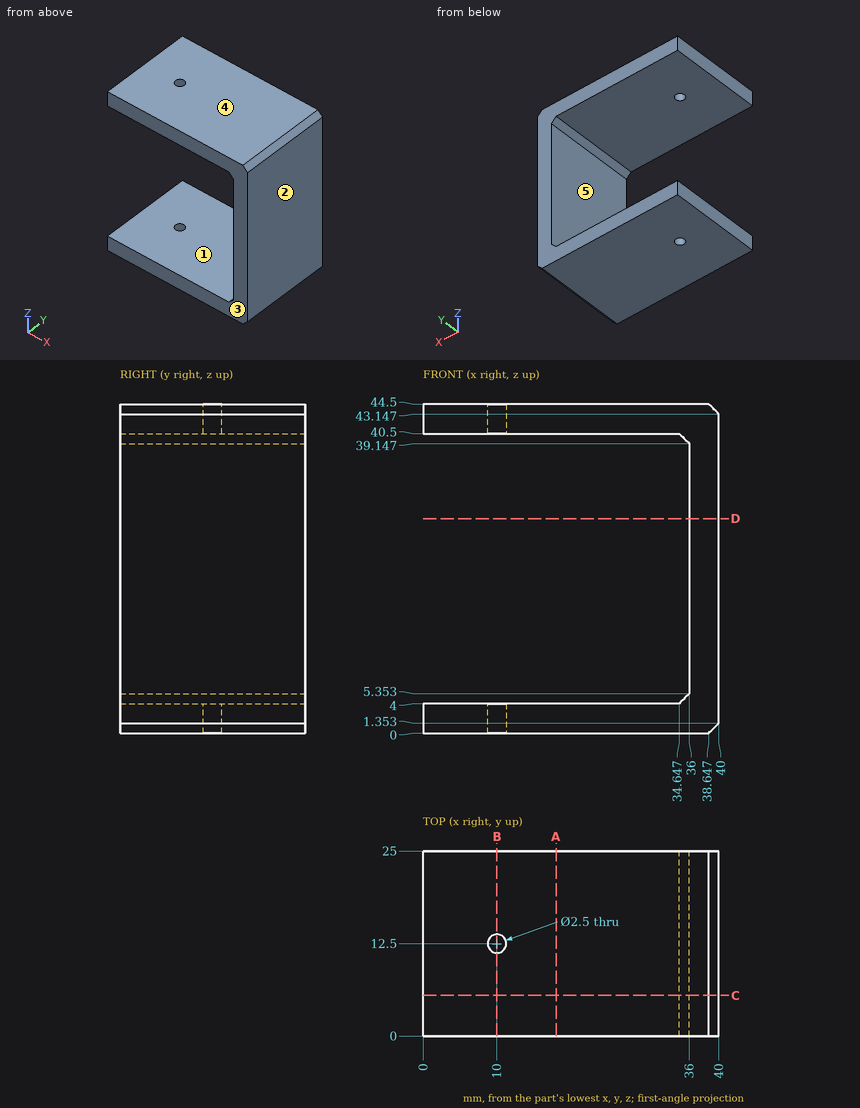
Verification items for this drawing (mm, ordinates from the low corner). A direction names the side the tool comes from. Give positions to 0.01 mm unless a question says otherwise; leave off trailing zeros. Write each loop counter-clockwise with the first axis right and the second up, starting at its lowest first coordinate (ties: lowest second). Pieces come first, ordered by that corner, then holes. Notation, with made-up numbers: (15.5, 29.5) - (33.5, 29.5) arc R15 cw to (33.5, 53.5) - close; hole circle Ø10 at (67.25, 11). An arc over 180 degrees is marked (long way). Answer as CSV lines item,"result". Start each with the question number.
1. Draft check along Z on the marked faces 3, 4 and 5. Enter one of: pulls with the +Z half, pulls with the -Z half, needs draft (parallel to the pull), parting line crosses it, or undercut.
2. Set-up check for the marked faces 1 and 2: record each of +Z, -Z, +X, -X, +Y, -Y from which the full face is reachable in a straight line by a thin tool's end or side.
3. Sectioned sample at C-C (y = 5.5). Record the boundary of the cut face in (x, z).
4. Thickness scan on line 1 (Z direction, x = 8, y = 4.5); line 2 (Y direction, x = 10, z = 2.3); line 3 (X direction, y = 17.25, z = 36.5). Record the ranges inside material, lowest first.
5. Sectioned sample at B-B (x = 10). Record the boundary of the cut face in (y, z), then the cut area to 3 significant figures.
6. Depth check by flat-ended pin: pin 1 (8 mm diameter, centred on y = 9.5, z = 12.5, fed in from -X); pin 2 (10 mm diameter, centred on x = 30, z = 9.5, fed in from -Y). Enter the tip coordinate at first touch or a pass-through.
7. Sectioned sample at A-A (x = 18). Record the boundary of the cut face in (y, z).
8. Sectioned sample at D-D (z = 29). Record the boundary of the cut face in (x, y).
Derived:
1,face 3,"needs draft"
1,face 4,"pulls with the +Z half"
1,face 5,"undercut"
2,face 1,"-X, +Y, -Y"
2,face 2,"+Z, -Z, +X, +Y, -Y"
3,outline,"(0, 0) - (38.65, 0) - (40, 1.35) - (40, 43.15) - (38.65, 44.5) - (0, 44.5) - (0, 40.5) - (34.65, 40.5) - (36, 39.15) - (36, 5.35) - (34.65, 4) - (0, 4) - close"
4,line 1,"0 to 4, 40.5 to 44.5"
4,line 2,"0 to 11.25, 13.75 to 25"
4,line 3,"36 to 40"
5,outline,"(0, 0) - (11.25, 0) - (11.25, 4) - (0, 4) - close; (0, 40.5) - (11.25, 40.5) - (11.25, 44.5) - (0, 44.5) - close; (13.75, 0) - (25, 0) - (25, 4) - (13.75, 4) - close; (13.75, 40.5) - (25, 40.5) - (25, 44.5) - (13.75, 44.5) - close"
5,area,"180 mm²"
6,pin 1,"x = 36"
6,pin 2,"through"
7,outline,"(0, 0) - (25, 0) - (25, 4) - (0, 4) - close; (0, 40.5) - (25, 40.5) - (25, 44.5) - (0, 44.5) - close"
8,outline,"(36, 0) - (40, 0) - (40, 25) - (36, 25) - close"
